Here's how the part is built. I have some questions about the finished solid (model axes, mm). Face numbers are marked on the shaded views. A direction names the side the tool comes from. Round coordinates to 2 decimals unless told otherwise and drop trailing zeros. Order: outer loops, then holes, each group sorted by start corner. A loop starts at its lowest first (then second) coordinate and runs counter-clockwise, first axis right, second up. Notation, with made-up numbers: (41, 26) -> (46, 26) arc R24 cw to (46, 58) -> close; hole circle Ø6 at (32, 64.5). An arc over 180 degrees is marked (long way). Use a Markdown table: item, result. Add a question column.
(1) If I drill on probe 1 along Z at (x, y) = (-18, -8.25); probe 2 along Z at (x, y) = (-60.5, -10); probe 3 along X at (y, z) = (-9, -2.5), over which ranges is the centre line in solid material (lowest first)?
(2) Thinking about a two-plate mould opening in Z: for the marked faces 1, 2 and 3, which applies, pulls with the +Z half, pulls with the -Z half, needs draft (parallel to the pull), parting line crosses it, or undercut?
(3) I want a section at C-C, the plane y = -4.75. Please give me the cut outline in (x, z) (3 decimals).
(4) I want a section at A-A, the plane x = -57.5. Please give me the cut outline in (y, z).
(5) I want a section at B-B, the plane z = 24. Please give me the cut outline in (x, y).
(6) On a 3-axis mill with a long thin cutter (end or side, diameter ignored), from which of +Z, -Z, +X, -X, +Y, -Y can I reach the whole of each face in a straight line? I mean the marked faces 4 and 5. Say none if no direction works.
(7) I'm going to push flat-ended pins straight in: P1, Ø6, axis at y = -8, z = -19, coming from the -X side; P2, Ø4, axis at y = -1.5, z = 24.5, coming from the -X side; P3, Ø3, axis at y = -10, z = -2, coming from the -X side. Where does each tip first touch, or does it pass through?
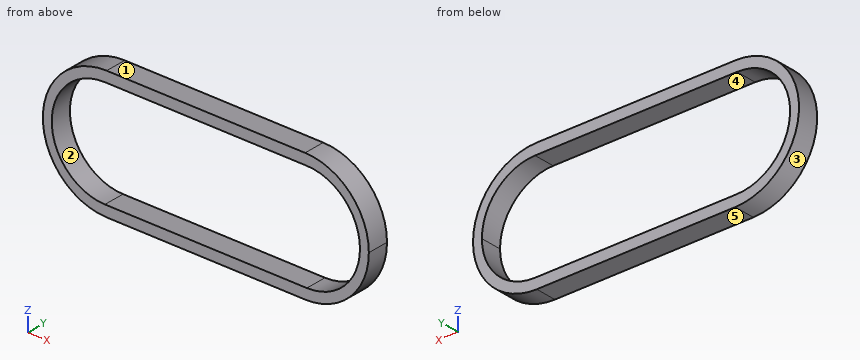
from build123d import *

# Parameters (mm, degrees)
F1_DEPTH = 12.7
F3_DEPTH = 25.4


with BuildPart() as f1:
    # F0 (on Front) → F1 (new body)
    with BuildSketch(Plane.XZ):
        with BuildLine():
            Line((-59.2836, 0), (-59.2836, 38.1))
            ThreePointArc((-59.2836, 38.1), (-97.3836, 0), (-59.2836, -38.1))
            Line((-59.2836, -38.1), (-59.2836, 0))
        make_face()
        with BuildLine():
            ThreePointArc((-21.1836, 0), (-32.342832, 26.940768), (-59.2836, 38.1))
            Line((-59.2836, 38.1), (-59.2836, 0))
            Line((-59.2836, 0), (-59.2836, -38.1))
            ThreePointArc((-59.2836, -38.1), (-32.342832, -26.940768), (-21.1836, 0))
        make_face()
        with BuildLine():
            Line((59.2836, 38.1), (-59.2836, 38.1))
            ThreePointArc((-59.2836, 38.1), (-32.342832, 26.940768), (-21.1836, 0))
            ThreePointArc((-21.1836, 0), (-32.342832, -26.940768), (-59.2836, -38.1))
            Line((-59.2836, -38.1), (59.2836, -38.1))
            ThreePointArc((59.2836, -38.1), (21.1836, 0), (59.2836, 38.1))
        make_face()
        with BuildLine():
            Line((59.2836, 0), (59.2836, 38.1))
            ThreePointArc((59.2836, 38.1), (21.1836, 0), (59.2836, -38.1))
            Line((59.2836, -38.1), (59.2836, 0))
        make_face()
        with BuildLine():
            ThreePointArc((97.3836, 0), (86.224368, 26.940768), (59.2836, 38.1))
            Line((59.2836, 38.1), (59.2836, 0))
            Line((59.2836, 0), (59.2836, -38.1))
            ThreePointArc((59.2836, -38.1), (86.224368, -26.940768), (97.3836, 0))
        make_face()
    extrude(amount=F1_DEPTH)

    # F2 (on Front) → F3 (cut)
    with BuildSketch(Plane.XZ):
        with BuildLine():
            Line((-60.325, 0), (-60.325, 31.75))
            ThreePointArc((-60.325, 31.75), (-92.075, 0), (-60.325, -31.75))
            Line((-60.325, -31.75), (-60.325, 0))
        make_face()
        with BuildLine():
            ThreePointArc((-28.575, 0), (-37.87436, 22.45064), (-60.325, 31.75))
            Line((-60.325, 31.75), (-60.325, 0))
            Line((-60.325, 0), (-60.325, -31.75))
            ThreePointArc((-60.325, -31.75), (-37.87436, -22.45064), (-28.575, 0))
        make_face()
        with BuildLine():
            ThreePointArc((60.325, -31.75), (28.575, 0), (60.325, 31.75))
            Line((60.325, 31.75), (-60.325, 31.75))
            ThreePointArc((-60.325, 31.75), (-37.87436, 22.45064), (-28.575, 0))
            ThreePointArc((-28.575, 0), (-37.87436, -22.45064), (-60.325, -31.75))
            Line((-60.325, -31.75), (60.325, -31.75))
        make_face()
        with BuildLine():
            Line((60.325, 0), (60.325, 31.75))
            ThreePointArc((60.325, 31.75), (28.575, 0), (60.325, -31.75))
            Line((60.325, -31.75), (60.325, 0))
        make_face()
        with BuildLine():
            ThreePointArc((92.075, 0), (82.77564, 22.45064), (60.325, 31.75))
            Line((60.325, 31.75), (60.325, 0))
            Line((60.325, 0), (60.325, -31.75))
            ThreePointArc((60.325, -31.75), (82.77564, -22.45064), (92.075, 0))
        make_face()
    extrude(amount=F3_DEPTH, mode=Mode.SUBTRACT)


solid = f1.part
Taken from the geometry:
| question | item | result |
|---|---|---|
| 1 | probe 1 | z = -38.1 to -31.75, 31.75 to 38.1 |
| 1 | probe 2 | z = -38.08 to -31.75, 31.75 to 38.08 |
| 1 | probe 3 | x = -97.3 to -91.98, 91.98 to 97.3 |
| 2 | face 1 | pulls with the +Z half |
| 2 | face 2 | undercut |
| 2 | face 3 | parting line crosses it |
| 3 | outline | (-59.284, -38.1) -> (59.284, -38.1) arc R38.1 ccw to (97.384, 0) arc R38.1 ccw to (59.284, 38.1) -> (-59.284, 38.1) arc R38.1 ccw to start; hole (-60.325, -31.75) -> (60.325, -31.75) arc R31.75 ccw to (92.075, 0) arc R31.75 ccw to (60.325, 31.75) -> (-60.325, 31.75) arc R31.75 ccw to start |
| 4 | outline | (-12.7, -38.1) -> (0, -38.1) -> (0, -31.75) -> (-12.7, -31.75) -> close; (-12.7, 31.75) -> (0, 31.75) -> (0, 38.1) -> (-12.7, 38.1) -> close |
| 5 | outline | (-88.87, -12.7) -> (-81.11, -12.7) -> (-81.11, 0) -> (-88.87, 0) -> close; (81.11, -12.7) -> (88.87, -12.7) -> (88.87, 0) -> (81.11, 0) -> close |
| 6 | face 4 | +Y, -Y |
| 6 | face 5 | -Z, +X, -X, +Y, -Y |
| 7 | P1 | stops at x = -93.86 |
| 7 | P2 | stops at x = -90.03 |
| 7 | P3 | stops at x = -97.38 |
